For this review, take the finished solid that the model builds, in its own axes (mm). A direction names the side the tool comes from. Round coordinates to 2 decimals unless told otherwise and drop trailing zeros. Loops run counter-clockwise (first coordinate to the right, second up) from the corner with the lowest first, then second, coordinate; pieces in that order, holes last. Notation, with made-up numbers: M 77.5,36.25 L 95.5,36.25 A17 cw 95.5,68.25 Z; hole C -26.75,84.25 d6. An arc over 180 degrees is marked long. One line per question, with ' | ' between items. Start each with the question number.
1) We need section C-C (z = 37). Give the boundary of the cut face in (x, y).
2) We need section A-A (x = -20). Give the boundary of the cut face in (y, z).
3) Mouldability with a two-part tool opening along Z and no side actions: class faces 1 (the face through (-15, 3, 33.656)), 2 (the face through (-17, 6, 25)), 3 (the face through (-25, 5, 0)), 4 (the face through (-6.22, 2.96, 30.77)) as pulls with the +Z half, pulls with the -Z half, needs draft (parallel to the pull), parting line crosses it, or undercut.
4) For pin 1 Ø16.5 at (x, z) = (-24, 14.5) entering from +Y; pin 2 Ø12 at (y, z) = (16, 35) entering from +X, all flat-tipped, find the tip position at first contact; note any pin that passes through.
5) For faces 5 (the face through (-33, 18, 25)), 6 (the face through (0, 3, 25)), 7 (the face through (-24.23, 2.96, 13.63)), list the 3-axis set-ups (+Z, -Z, +X, -X, +Y, -Y) from which the entire face can be reached by the end or side of a thin tool; tool diameter is ignored.
6) We need section B-B (z = 30.7). Give the boundary of the cut face in (x, y), and give its area (3 significant figures).
7) We need section D-D (y = 20.5). Give the boundary of the cut face in (x, z), and give its area (3 significant figures).
8) For probe 1 along X at (y, z) = (9.25, 20.5); probe 2 along Y at (x, z) = (-23.5, 28); probe 3 along Z at (x, y) = (-6.5, 4.25), list the stretches that pass through material, from the lowest coordinate up. Write a range as from..to.
```python
from build123d import *

# Parameters (mm, degrees)
BOSS_EXTRUDE1_DEPTH = 50
CUT_EXTRUDE1_DEPTH  = 14


with BuildPart() as part:
    # Sketch1 → Boss-Extrude1 (new body)
    with BuildSketch(Plane.XY):
        Polygon((0, 0), (-39, 0), (-39, 30), (-33, 30), (-33, 6), (0, 6), align=None)
    extrude(amount=BOSS_EXTRUDE1_DEPTH)

    # Sketch2 → Cut-Extrude1 (cut)
    with BuildSketch(Plane.XZ):
        with BuildLine():
            Line((-21.273396894, 33.65603272), (-9.173396894, 33.65603272))
            ThreePointArc((-9.173396894, 33.65603272), (-6.217364174, 30.7), (-9.173396894, 27.74396728))
            Line((-9.173396894, 27.74396728), (-21.273396894, 27.74396728))
            ThreePointArc((-21.273396894, 27.74396728), (-24.229429614, 30.7), (-21.273396894, 33.65603272))
        make_face()
        with BuildLine():
            Line((-21.273396894, 16.65603272), (-9.173396894, 16.65603272))
            ThreePointArc((-9.173396894, 16.65603272), (-6.217364174, 13.7), (-9.173396894, 10.74396728))
            Line((-9.173396894, 10.74396728), (-21.273396894, 10.74396728))
            ThreePointArc((-21.273396894, 10.74396728), (-24.229429614, 13.7), (-21.273396894, 16.65603272))
        make_face()
    extrude(amount=-CUT_EXTRUDE1_DEPTH, mode=Mode.SUBTRACT)


solid = part.part
```
Answers below:
1) outline: M -39,0 L 0,0 L 0,6 L -33,6 L -33,30 L -39,30 Z
2) outline: M 0,0 L 6,0 L 6,10.74 L 0,10.74 Z; M 0,16.66 L 6,16.66 L 6,27.74 L 0,27.74 Z; M 0,33.66 L 6,33.66 L 6,50 L 0,50 Z
3) face 1: undercut | face 2: needs draft | face 3: pulls with the -Z half | face 4: undercut
4) pin 1: y = 6 | pin 2: x = -33
5) face 5: +Z, -Z, +X, +Y | face 6: +Z, -Z, +X, +Y, -Y | face 7: +Y, -Y
6) outline: M -39,0 L -24.23,0 L -24.23,6 L -33,6 L -33,30 L -39,30 Z; M -6.22,0 L 0,0 L 0,6 L -6.22,6 Z | area: 270 mm^2
7) outline: M -39,0 L -33,0 L -33,50 L -39,50 Z | area: 300 mm^2
8) probe 1: -39..-33 | probe 2: 0..6 | probe 3: 0..12.44, 14.96..29.44, 31.96..50
